from build123d import *

# Parameters (mm, degrees)
SALIENTE_EXTRUIR2_DEPTH = 5
CROQUIS4_W              = 3
CROQUIS4_H              = 6
CORTAR_EXTRUIR1_DEPTH   = 4


with BuildPart() as part:
    # Croquis2 → Saliente-Extruir2 (new body)
    with BuildSketch(Plane(origin=(0, 0, 0), x_dir=(0, 0, -1), z_dir=(1, 0, 0))):
        Polygon((0, 3), (4, -1), (4, -3), (-4, -3), (-4, 3), align=None)
    extrude(amount=SALIENTE_EXTRUIR2_DEPTH)

    # Croquis4 → Cortar-Extruir1 (cut)
    with BuildSketch(Plane(origin=(0, 3, 0), x_dir=(1, 0, 0), z_dir=(0, 1, 0))):
        with Locations((3.5, 1)):
            Rectangle(CROQUIS4_W, CROQUIS4_H)
    extrude(amount=-CORTAR_EXTRUIR1_DEPTH, mode=Mode.SUBTRACT)


solid = part.part
Geometry: final body of the model. Coordinates: model frame, mm. A direction names the side the tool comes from. Round coordinates to 2 decimals unless told otherwise and drop trailing zeros. Loops run counter-clockwise (first coordinate to the right, second up) from the corner with the lowest first, then second, coordinate; pieces in that order, holes last.
Q1. Section C-C on x = 1.3. Return loops of the section in (y, z), plus the area to 3 significant figures.
Q2. Section B-B on x = 4.5. Return loops of the section in (y, z), plus the area to 3 significant figures.
Q3. Access query for faces 1 (the flat face through (2, 0, 4)), 2 (the flat face through (3, -1, -1)). Directions: +Z, -Z, +X, -X, +Y, -Y. A direction counts if a zero-diameter tool reaches every point of the face in a straight line with its end or side. Return the directions, or none.
Q4. Material intervals for L1, parallel to X at y = 0.25, z = -1.75; L2, parallel to Z at x = 3.85, y = 0.2; L3, parallel to Y at x = 0.5, z = -2.25, sorted ascending.
Q5. Section A-A on y = 1.6. Return loops of the section in (x, z), plus the area to 3 significant figures.
Q6. Pin query (flat end, axial travel): P1, Ø2, axis at y = 1.5, z = 0, coming from the +X side; P2, Ø0.9, axis at x = 3, z = 0, coming from the +Y side. Return the tip coordinate at first contact, or that it passes through.
Evaluation:
1. outline: (-3, -4) - (-1, -4) - (3, 0) - (3, 4) - (-3, 4) - close
1. area: 40.0 mm2
2. outline: (-3, -4) - (-1, -4) - (-1, 2) - (3, 2) - (3, 4) - (-3, 4) - close
2. area: 24.0 mm2
3. face 1: +Z, +X, -X, +Y, -Y
3. face 2: -Z, +X, +Y
4. L1: x = 0 to 2
4. L2: z = 2 to 4
4. L3: y = -3 to 0.75
5. outline: (0, -1.4) - (2, -1.4) - (2, 2) - (5, 2) - (5, 4) - (0, 4) - close
5. area: 16.8 mm2
6. P1: stops at x = 2
6. P2: stops at y = -1
